Print and shaded views of the part. All mm, measured from the part's lowest x, y and z. Round coordinates to 2 decimals unless told otherwise and drop trailing zeros. Write each loop counter-clockwise with the first axis right and the second up, starting at its lowest first coordinate (ties: lowest second). Pieces come first, ordered by that corner, then holes. Notation, with made-up numbers: (57, 10.25) - (64, 10.25) arc R8 cw to (64, 16.25) - close; hole circle Ø6 at (44.25, 67). An arc over 180 degrees is marked (long way). One line per item, written item: value.
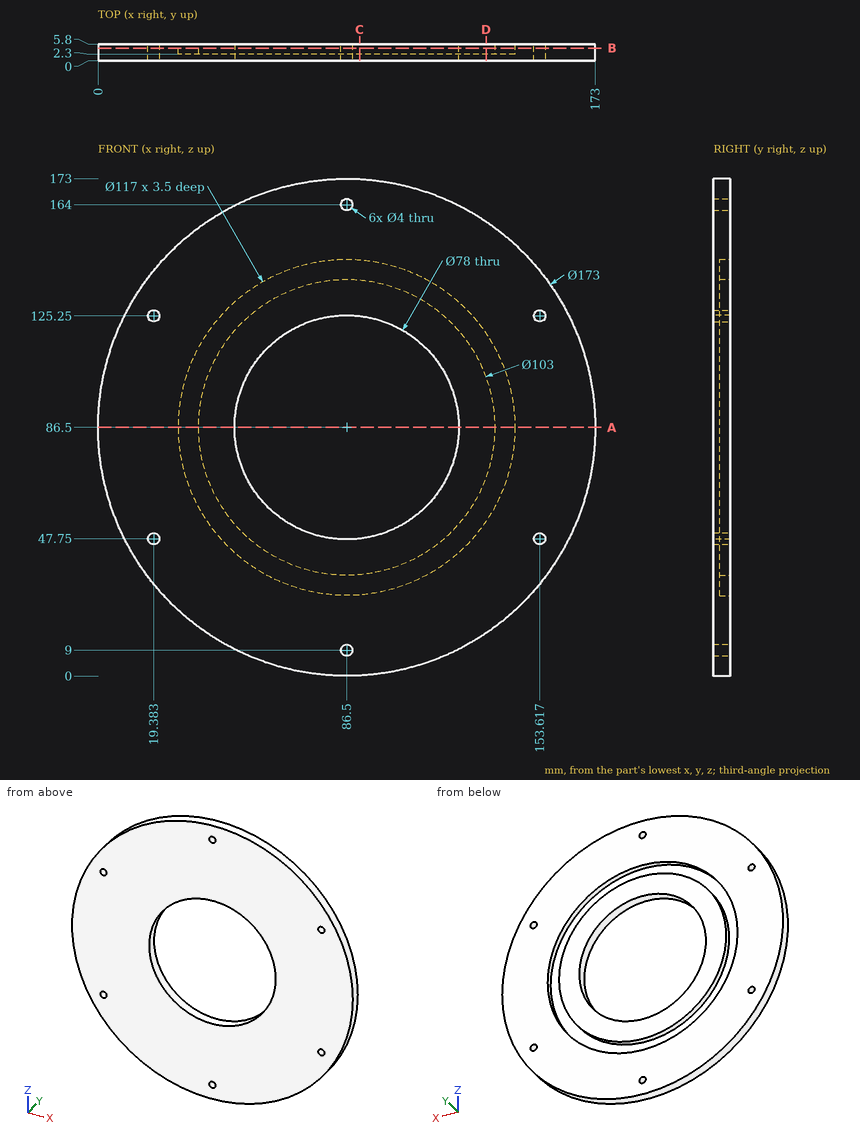
1. Band-saw the part on A-A on z = 86.5. Write the cut outline in (x, y).
Report:
outline: (0, 0) - (47.5, 0) - (47.5, 5.8) - (35, 5.8) - (35, 2.3) - (28, 2.3) - (28, 5.8) - (0, 5.8) - close; (125.5, 0) - (173, 0) - (173, 5.8) - (145, 5.8) - (145, 2.3) - (138, 2.3) - (138, 5.8) - (125.5, 5.8) - close
2. Drop flat-ended pins along their axis: pin 1 (3 mm diameter, centred on x = 153.62, z = 125.25, fed in from +Y); pin 2 (1 mm diameter, centred on x = 46.5, y = 3, fed in from -Z); pin 3 (1.5 mm diameter, centred on x = 46.5, y = 5, fed in from -Z); pin 4 (3 mm diameter, centred on x = 74, y = 2.5, fed in from -Z). Give the stop position or say it passes through.
Report:
pin 1: through
pin 2: z = 9.55
pin 3: z = 9.42
pin 4: z = 0.7
3. Wall check: probe 1 along X at (y, z) = (3.15, 86.5); probe 2 along Z at (x, y) = (86.5, 1.9); probe 3 along Z at (x, y) = (86.5, 4). Give the ranges that are in metal, low to high. Write a range as [from, to].
Report:
probe 1: [0, 28], [35, 47.5], [125.5, 138], [145, 173]
probe 2: [0, 7], [11, 47.5], [125.5, 162], [166, 173]
probe 3: [0, 7], [11, 28], [35, 47.5], [125.5, 138], [145, 162], [166, 173]
4. Band-saw the part on D-D on x = 135. Write the cut outline in (y, z).
Report:
outline: (0, 14.88) - (5.8, 14.88) - (5.8, 53.79) - (2.3, 53.79) - (2.3, 69.18) - (5.8, 69.18) - (5.8, 103.82) - (2.3, 103.82) - (2.3, 119.21) - (5.8, 119.21) - (5.8, 158.12) - (0, 158.12) - close
5. Band-saw the part on C-C on x = 91. Write the cut outline in (y, z), plus the area to 4 significant figures.
Report:
outline: (0, 0.12) - (5.8, 0.12) - (5.8, 28.17) - (2.3, 28.17) - (2.3, 35.2) - (5.8, 35.2) - (5.8, 47.76) - (0, 47.76) - close; (0, 125.24) - (5.8, 125.24) - (5.8, 137.8) - (2.3, 137.8) - (2.3, 144.83) - (5.8, 144.83) - (5.8, 172.88) - (0, 172.88) - close
area: 503.5 mm²
6. Band-saw the part on B-B on y = 4.4. State how many separate pieces and enclosed holes the cut face has, plus the area to 3 significant figures.
Report:
separate pieces: 2
enclosed holes: 8
area: 16,200 mm²
